The model under review builds one solid part; all positions refer to its coordinate system, in mm. Face numbers are marked on the shaded views. A direction names the side the tool comes from. Give positions to 0.01 mm unless a question says otherwise; leave off trailing zeros. Write each loop counter-clockwise with the first axis right and the second up, starting at its lowest first coordinate (ties: lowest second). Pieces come first, ordered by that corner, then holes. Notation, with made-up numbers: M 63,13 L 82,13 A15 ccw 82,35 Z; hole C -14,-34.75 d10. An arc over 180 degrees is marked long. Write item = value, one per line. Start each with the question number.
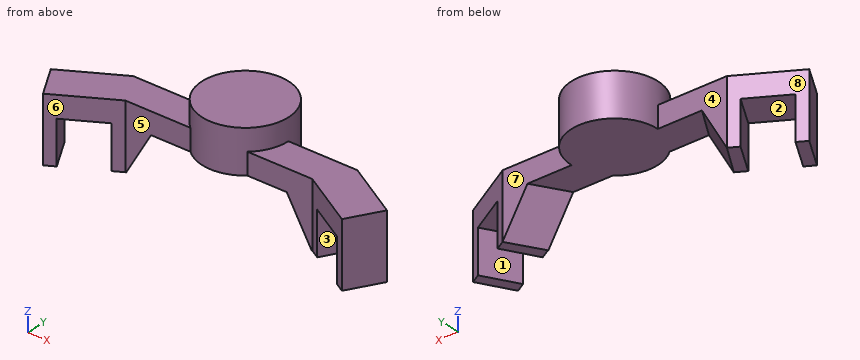
```python
from build123d import *

# Parameters (mm, degrees)
PAD001_DEPTH = 10
PAD_DEPTH    = 30
SKETCH001_W  = 20
SKETCH001_H  = 20
POCKET_DEPTH = 50


with BuildPart() as loft_body:
    # Sketch002 → Loft section 0
    with BuildSketch(Plane.XZ.offset(-85)):
        Polygon((1, 20), (-31.452995, 20), (-43, 0), (1, 0), align=None)
    # Sketch003 → Loft section 1
    with BuildSketch(Plane(origin=(0, 100, 0), x_dir=(-1, 0, 0), z_dir=(0, 1, 0))):
        Polygon((0, 20), (40.452995, 20), (52, 0), (0, 0), align=None)
    loft()


with BuildPart() as pad001:
    # Sketch005 → Pad001 (new body, symmetric)
    with BuildSketch(Plane.XY.offset(30)):
        with BuildLine():
            ThreePointArc((0, 120), (-20, 100), (0, 80))
            Line((0, 120), (0, 80))
        make_face()
    extrude(amount=PAD001_DEPTH, both=True)


with BuildPart() as cut:
    # Sketch → Pad (new body)
    with BuildSketch(Plane.XY):
        Polygon((-51.961524, 100), (0, 100), (0.112312, 85), (-43.30127, 85), (-69.282032, 70), (-77.942286, 85), align=None)
    extrude(amount=PAD_DEPTH)

    # Sketch001 → Pocket (cut)
    with BuildSketch(Plane(origin=(-47.631397, 82.5, 0), x_dir=(0.866025, 0.5, 0), z_dir=(0.5, -0.866025, 0))):
        with Locations((-10, 10)):
            Rectangle(SKETCH001_W, SKETCH001_H)
    extrude(amount=-POCKET_DEPTH, mode=Mode.SUBTRACT)

    # Fusion: union Pad001
    add(pad001.part)

    # Cut: cut Loft body
    add(loft_body.part, mode=Mode.SUBTRACT)


with BuildPart() as fusion001:
    # Part__Mirroring: instance of Cut
    add(cut.part.mirror(Plane(origin=(0, 0, 0), x_dir=(0, -1, 0), z_dir=(1, 0, 0))))

    # Fusion001: union Cut
    add(cut.part)


solid = fusion001.part
```
Item 1: We need section A-A, the plane y = 78. Write out the cut boundary in (x, z).
Item 2: Clearance check with flat-ended pins moving along their axes: P1, Ø10, axis at x = -13, z = 23.5, coming from the +Y side; P2, Ø24, axis at x = -39, z = 22.5, coming from the +Y side; P3, Ø3, axis at y = 80, z = 32.5, coming from the +X side; P4, Ø5, axis at x = 39, z = 33, coming from the +Y side. State where each tip first meets the part, or that it passes through.
Item 3: The part is to be moulded in two halves that separate along X. For the marked faces 6, 7 and 8, say which applies: released by +X, released by -X, zero draft, split by the parting line, or undercut.
Item 4: We need section D-D, the plane z = 18. Give the number of separate pieces and of enclosed holes in the cut face, and give its area (3 significant figures).
Item 5: For the marked faces 1, 2, 3, 4 and 5, list the 3-axis set-ups (+Z, -Z, +X, -X, +Y, -Y) from which the entire face can be reached by the end or side of a thin tool; tool diameter is ignored.
Item 6: We need section B-B, the plane z = 26. Write out the cut boundary in (x, y).
Item 7: We need section C-C, the plane x = 0. Write out the cut boundary in (y, z).
Item 8: To check wall thickness, follow probe 1 along Z at (x, y) = (29.5, 95.5); probe 2 along X at (y, z) = (84, 14.5); probe 3 along X at (y, z) = (90.5, 8). State the ranges of each line that lie inside material, in increasing order. Write a range as [from, to].
Worked out:
q1.outline = M -73.9,0 L -68.13,0 L -68.13,20 L -55.43,20 L -55.43,30 L -73.9,30 Z; M 55.43,20 L 68.13,20 L 68.13,0 L 73.9,0 L 73.9,30 L 55.43,30 Z
q2.P1 = 118.33
q2.P2 = 100
q2.P3 = 7.6
q2.P4 = through
q3.face_6 = undercut
q3.face_7 = zero draft
q3.face_8 = released by -X
q4.separate_pieces = 4
q4.enclosed_holes = 0
q4.area = 662 mm²
q5.face_1 = -Z, +Y
q5.face_2 = -Z
q5.face_3 = -Z, -Y
q5.face_4 = +Z, -Z, -X, +Y
q5.face_5 = +Z, -Z, -Y
q6.outline = M -77.94,85 L -69.28,70 L -43.3,85 L -13.23,85 A20 ccw 13.23,85 L 43.3,85 L 69.28,70 L 77.94,85 L 51.96,100 L 20,100 A20 ccw -20,100 L -51.96,100 Z
q7.outline = M 80,20 L 120,20 L 120,40 L 80,40 Z
q8.probe_1 = [20, 30]
q8.probe_2 = [-77.36, -71.59], [-48.5, -45.03], [45.03, 48.5], [71.59, 77.36]
q8.probe_3 = [-52.25, -41.68], [41.68, 52.25]
